from build123d import *

# Parameters (mm, degrees)
BOSS_EXTRUDE1_DEPTH = 10
SKETCH2_R           = 22
CUT_EXTRUDE1_DEPTH  = 10


with BuildPart() as part:
    # Sketch1 → Boss-Extrude1 (new body)
    with BuildSketch(Plane(origin=(0, 0, 0), x_dir=(1, 0, 0), z_dir=(0, 1, 0))):
        with BuildLine():
            Line((224.059047254, 44.109057501), (-188.882980363, 44.109057501))
            Line((-188.882980363, 44.109057501), (-201.155616653, 16.794241143))
            ThreePointArc((-201.155616653, 16.794241143), (-201.308951392, 13.078635624), (-198.854573143, 10.28484549))
            Line((-198.854573143, 10.28484549), (-28.764010839, -75.890942499))
            Line((-28.764010839, -75.890942499), (17.588033446, -75.890942499))
            Line((17.588033446, -75.890942499), (63.94007773, -75.890942499))
            Line((63.94007773, -75.890942499), (234.030640034, 10.28484549))
            ThreePointArc((234.030640034, 10.28484549), (236.485018284, 13.078635624), (236.331683544, 16.794241143))
            Line((236.331683544, 16.794241143), (224.059047254, 44.109057501))
        make_face()
    extrude(amount=BOSS_EXTRUDE1_DEPTH)

    # Sketch2 → Cut-Extrude1 (cut)
    with BuildSketch(Plane(origin=(0, 10, 0), x_dir=(1, 0, 0), z_dir=(0, 1, 0))):
        with Locations(Location((17.588033446, -15.890942499, 0), (0, 0, 270))):
            Circle(SKETCH2_R)
    extrude(amount=-CUT_EXTRUDE1_DEPTH, mode=Mode.SUBTRACT)


solid = part.part
Geometry check sheet. Reference: the model listing, model coordinates, mm. Round coordinates to 2 decimals unless told otherwise and drop trailing zeros. Order: outer loops, then holes, each group sorted by start corner. A loop starts at its lowest first (then second) coordinate and runs counter-clockwise, first axis right, second up. Notation, with made-up numbers: (-8, 66.25) - (38, 66.25) arc R15 ccw to (38, 78.25) - close; hole circle Ø10 at (-32, 89). An arc over 180 degrees is marked (long way). One line per question, with ' | ' between items. Start each with the question number.
(1) Thickness scan on L1, parallel to X at y = 2.25, z = 30; L2, parallel to X at y = 9.25, z = 24.5; L3, parallel to Z at x = 24, y = 6.25. Record the ranges inside material, lowest first. Write a range as [from, to].
(2) Release check for a two-part mould opening along Z. For faces 1 (the flat face through (15, 0, -12)), 2 (the flat face through (230.28, 4.93, -30.26)), 3 (the cylindrical face through (-3.89, 5.07, 11.12)) record: released by +Z, released by -Z, zero draft, split by the parting line, or undercut.
(3) Sectioned sample at C-C on y = 7.5. Record the cut outline in (x, z), and give its area (3 significant figures).
(4) Sectioned sample at B-B on x = 6. Record the cut outline in (y, z), and give its area (3 significant figures).
(5) Sectioned sample at A-A on z = 17. Record the cut outline in (x, y), and give its area (3 significant figures).
(6) Depth check by flat-ended pin: pin 1 Ø2 at (y, z) = (6, 24) entering from +X; pin 2 Ø3 at (x, z) = (-146.5, 19) entering from +Y; pin 3 Ø4 at (y, z) = (2, 42.5) entering from -X. Enter the tip coordinate at first touch or a pass-through.
(7) Sectioned sample at D-D on x = -56. Record the cut outline in (y, z).
Conclusion:
1) L1: x = [-119.34, 0.71], [34.47, 154.52] | L2: x = [-130.2, -2.66], [37.83, 165.37] | L3: z = [-44.11, -5.15], [36.94, 75.89]
2) face 1: zero draft | face 2: released by -Z | face 3: undercut
3) outline: (-201.16, -16.79) - (-188.88, -44.11) - (224.06, -44.11) - (236.33, -16.79) arc R5 ccw to (234.03, -10.28) - (63.94, 75.89) - (-28.76, 75.89) - (-198.85, -10.28) arc R5 ccw to start; hole circle Ø44 at (17.59, 15.89) | area: 35,600 mm2
4) outline: (0, -44.11) - (10, -44.11) - (10, -2.81) - (0, -2.81) - close; (0, 34.59) - (10, 34.59) - (10, 75.89) - (0, 75.89) - close | area: 826 mm2
5) outline: (-145, 0) - (-4.38, 0) - (-4.38, 10) - (-145, 10) - close; (39.56, 0) - (180.18, 0) - (180.18, 10) - (39.56, 10) - close | area: 2,810 mm2
6) pin 1: stops at x = 168.33 | pin 2: passes through | pin 3: stops at x = -98.62
7) outline: (0, -44.11) - (10, -44.11) - (10, 62.09) - (0, 62.09) - close
